```python
from build123d import *

# Parameters (mm, degrees)
EXTRUDE_1_DEPTH     = 22.67
SKETCH_3_R          = 3.65
CUT_EXTRUDE_1_DEPTH = 22.67
SKETCH_7_R          = 2.5
EXTRUDE_2_DEPTH     = 45
SKETCH_8_R          = 12.5
EXTRUDE_3_DEPTH     = 52


with BuildPart() as part:
    # 草图1 → 凸台-拉伸1 (new body)
    with BuildSketch(Plane.XY):
        with BuildLine():
            Line((-31.5, 35.5), (-14.5, 35.5))
            ThreePointArc((-14.5, 35.5), (0, 21), (-14.5, 6.5))
            Line((-14.5, 6.5), (-31.5, 6.5))
            ThreePointArc((-31.5, 6.5), (-46, 21), (-31.5, 35.5))
        make_face()
    extrude(amount=EXTRUDE_1_DEPTH)

    # 草图3 → 切除-拉伸1 (cut)
    with BuildSketch(Plane(origin=(0, 0, 0), x_dir=(-1, 0, 0), z_dir=(0, 0, -1))):
        with Locations((31.5, 11)):
            Circle(SKETCH_3_R)
        with Locations((31.5, 31)):
            Circle(SKETCH_3_R)
        with Locations((41.5, 21)):
            Circle(SKETCH_3_R)
    extrude(amount=-CUT_EXTRUDE_1_DEPTH, mode=Mode.SUBTRACT)

    # 草图7 → 凸台-拉伸2 (add)
    with BuildSketch(Plane(origin=(0, 0, 0), x_dir=(-1, 0, 0), z_dir=(0, 0, -1))):
        with Locations(Location((31.5, 21, 0), (0, 0, 180))):
            Circle(SKETCH_7_R)
    extrude(amount=EXTRUDE_2_DEPTH)

    # 草图8 → 凸台-拉伸3 (add)
    with BuildSketch(Plane.XY.offset(22.67)):
        with Locations(Location((-14.5, 21, 0), (0, 0, 180))):
            Circle(SKETCH_8_R)
    extrude(amount=EXTRUDE_3_DEPTH)


solid = part.part
```
The model under review builds one solid part; all positions refer to its coordinate system, in mm. A direction names the side the tool comes from. Give positions to 0.01 mm unless a question says otherwise; leave off trailing zeros. Order: outer loops, then holes, each group sorted by start corner. A loop starts at its lowest first (then second) coordinate and runs counter-clockwise, first axis right, second up. Notation, with made-up numbers: (-38.5, 79) - (8.5, 79) arc R31 ccw to (8.5, 104) - close; hole circle Ø11 at (-30.75, 7). An arc over 180 degrees is marked (long way). Use CSV: the item, a comma, the result in double quotes. Start each with the question number.
Q1. The part is to be moulded in two halves that separate along Y. For faces 1 (the cylindrical face through (-34, 21, -22)), 2 (the cylindrical face through (-28.603, 8.779, 11.176)), 3 (the flat face through (-23, 21, 0)), say which applies: +Y half, -Y half, draft (parallel to the pull), parting line (faces both ways), or undercut.
Q2. We need section A-A, the plane y = 11. Write out the cut boundary in (x, z), and give its area (3 significant figures).
Q3. We need section D-D, the plane y = 21. Write out the cut boundary in (x, z).
Q4. Clearance check with flat-ended pins moving along their axes: pin 1 Ø6 at (x, y) = (-40.5, 32) entering from +Z; pin 2 Ø10 at (y, z) = (32, 17) entering from +X; pin 3 Ø5 at (x, y) = (-20.5, 12.5) entering from -Z. State where each tip first meets the part, or that it passes through.
Q5. We need section C-C, the plane x = -22. Write out the cut boundary in (y, z).
Q6. We need section B-B, the plane x = -41.5. Write out the cut boundary in (y, z), and give its area (3 significant figures).
Q7. To check wall thickness, follow line 1 along Y through (x, z) = (-31.5, 12.5); line 2 along Z through (x, y) = (-36, 7.75); line 3 along Z through (x, y) = (-16.5, 21.5). State the ranges of each line that lie inside material, in increasing order. Write a range as [from, to].
Q8. Tool access review of faces 4 (the cylindrical face through (-4.58, 28.606, 48.306)), 5 (the cylindrical face through (-28.603, 28.779, 11.176)): name each direction out of +Z, -Z, +X, -X, +Y, -Y from which nothing blocks a thin tool from reaching the whole face with its end or side.
Outcome:
1,face 1,"parting line"
1,face 2,"undercut"
1,face 3,"draft"
2,outline,"(-42, 0) - (-35.15, 0) - (-35.15, 22.67) - (-42, 22.67) - close; (-27.85, 0) - (-4, 0) - (-4, 22.67) - (-7, 22.67) - (-7, 74.67) - (-22, 74.67) - (-22, 22.67) - (-27.85, 22.67) - close"
2,area,"1,480 mm^2"
3,outline,"(-46, 0) - (-45.15, 0) - (-45.15, 22.67) - (-46, 22.67) - close; (-37.85, 0) - (-34, 0) - (-34, -45) - (-29, -45) - (-29, 0) - (0, 0) - (0, 22.67) - (-2, 22.67) - (-2, 74.67) - (-27, 74.67) - (-27, 22.67) - (-37.85, 22.67) - close"
4,pin 1,"stops at z = 22.67"
4,pin 2,"stops at x = -1.3"
4,pin 3,"stops at z = 0"
5,outline,"(6.5, 0) - (35.5, 0) - (35.5, 22.67) - (31, 22.67) - (31, 74.67) - (11, 74.67) - (11, 22.67) - (6.5, 22.67) - close"
6,outline,"(10.5, 0) - (17.35, 0) - (17.35, 22.67) - (10.5, 22.67) - close; (24.65, 0) - (31.5, 0) - (31.5, 22.67) - (24.65, 22.67) - close"
6,area,"311 mm^2"
7,line 1,"y = [6.5, 7.35], [14.65, 27.35], [34.65, 35.5]"
7,line 2,"z = [0, 22.67]"
7,line 3,"z = [0, 74.67]"
8,face 4,"+Z"
8,face 5,"+Z, -Z"
